Autodesk Inventor part; units mm, degrees
ref_plane "YZ Plane" through (0, 0, 0) normal (1, 0, 0) x (0, 1, 0)
ref_plane "XZ Plane" through (0, 0, 0) normal (0, 1, 0) x (-1, 0, 0)
ref_plane "XY Plane" through (0, 0, 0) normal (0, 0, 1) x (1, 0, 0)
sketch "Sketch1" plane through (0, 0, 0) normal (0, 1, 0) x (-1, 0, 0)
  line L0 (659.75, 765) -> (-659.75, 765)
  line L1 (-659.75, 765) -> (-659.75, -765)
  line L2 (-659.75, -765) -> (659.75, -765)
  line L3 (659.75, -765) -> (659.75, 765)
  line L4 (659.75, 765) -> (-659.75, -765) construction
  line L5 (-659.75, 765) -> (659.75, -765) construction
  point P0 (0, 0)
  dimension "d0" = 1319.5
  dimension "d1" = 1530
extrude "Plate1" add sketch "Sketch1" along normal blind 2
sketch "Sketch2" plane through (0, 2, 0) normal (0, 1, 0) x (1, 0, 0)
  line L0 (-108.25, -435) -> (-108.25, 765)
  line L1 (-108.25, -430.2912) -> (661.75, -217.4503)
  line L2 (659.75, -765) -> (-659.75, -765)
  line L3 (659.75, 765) -> (659.75, -765)
  line L4 (-659.75, 765) -> (659.75, 765)
  line L5 (-659.75, -765) -> (-659.75, 765)
  point P0 (0, 0)
  point P1 (659.75, -218.0031)
extrude "Extrusion1" cut sketch "Sketch2" against normal through all contours L0 L4 L3 L1
equation "\"d2\" = Thickness"
equation "\"BendRadius\" = Thickness"
equation "\"BendReliefWidth\" = Thickness"
equation "\"BendReliefDepth\" = 0.5 * Thickness"
equation "\"CornerReliefSize\" = 4 * Thickness"
equation "\"MinimumRemnant\" = 2 * Thickness"
equation "\"TransitionRadius\" = BendRadius"
equation "\"JacobiRadiusSize\" = BendRadius"
equation "\"GapSize\" = Thickness"
properties part number "Top"
Design review of the part built by this model. Coordinates are the model's own, in mm. Round coordinates to 2 decimals unless told otherwise and drop trailing zeros. Write each loop counter-clockwise with the first axis right and the second up, starting at its lowest first coordinate (ties: lowest second). Pieces come first, ordered by that corner, then holes. Notation, with made-up numbers: (60, -19.5) -> (89, -19.5) arc R10 cw to (89, -3.5) -> close; hole circle Ø4 at (68, -35.75). An arc over 180 degrees is marked (long way). One line per question, with ' | ' between items.
(1) Take a section at A-A, the plane y = 1.2. State the section outline as (x, z) points, and give its area (3 significant figures).
Result sheet:
outline: (-659.75, -765) -> (-108.25, -765) -> (-108.25, 430.29) -> (659.75, 218) -> (659.75, 765) -> (-659.75, 765) -> close | area: 1,180,000 mm2
(2) Draft analysis for pull direction X (two halves, no side actions). For faces 1 (the flat face through (270.374, 1.014, 325.633)), 2 (the flat face through (-137, 0, 181)), state which applies: released by +X, released by -X, zero draft, split by the parting line, or undercut.
Result sheet:
face 1: undercut | face 2: zero draft
(3) Wall thickness on line 1 (X direction, y = 1.15, z = -661.5); line 2 (Z direction, x = -80.5, y = 1.1); line 3 (Z direction, x = 360.5, y = 1.7): over which ranges is each line inside the solid? List them lowest first. Write a range as [from, to].
Result sheet:
line 1: [-659.75, -108.25] | line 2: [422.62, 765] | line 3: [300.72, 765]
(4) Insertion check: P1, Ø1, axis at y = 0.5, z = -396, coming from the +X side. The pin has a flat end and moves straight along its axis. Give the tip position at first contact, or say it passes through.
Result sheet:
P1: x = -108.25
(5) Take a section at C-C, the plane z = -481.5. State the section outline as (x, y) points.
Result sheet:
outline: (-659.75, 0) -> (-108.25, 0) -> (-108.25, 2) -> (-659.75, 2) -> close
(6) Take a section at B-B, the plane x = 525. State the section outline as (y, z) points.
Result sheet:
outline: (0, 255.25) -> (2, 255.25) -> (2, 765) -> (0, 765) -> close
